Build history of the part. All positions in model axes, mm. Face numbers are marked on the shaded views. A direction names the side the tool comes from. Coordinates: 2 decimals unless noted, no trailing zeros. Loops run counter-clockwise (first coordinate to the right, second up) from the corner with the lowest first, then second, coordinate; pieces in that order, holes last.
Item 1: 3-axis set-ups, long thin cutter, end or side, ignore diameter. For the marked faces 1, 2 and 3: which of +Z, -Z, +X, -X, +Y, -Y reach the whole face in a straight line?
Item 2: Cut at B-B (x = 59). List the corners of the cut face in (y, z).
Item 3: Cut at C-C (y = -60). List the corners of the cut face in (x, z), and give its area (3 significant figures).
Item 4: Cut at A-A (z = 22). List the corners of the cut face in (x, y).
Item 5: Flat gauge pins, fed straight in: pin 1 (16.5 mm diameter, centred on x = 82, y = 57, fed in from +Z); pin 2 (9 mm diameter, centred on x = -5.5, z = 12, fed in from +Y); pin 3 (15 mm diameter, centred on x = 54, z = 12, fed in from -Y). Where does each tip first touch, or does it go through?
Item 6: Drill centre lines: line 1 along Y through (x, z) = (136, 21); line 2 along Z through (x, y) = (-18, 33.5). Where is each one in solid material? Low to high.
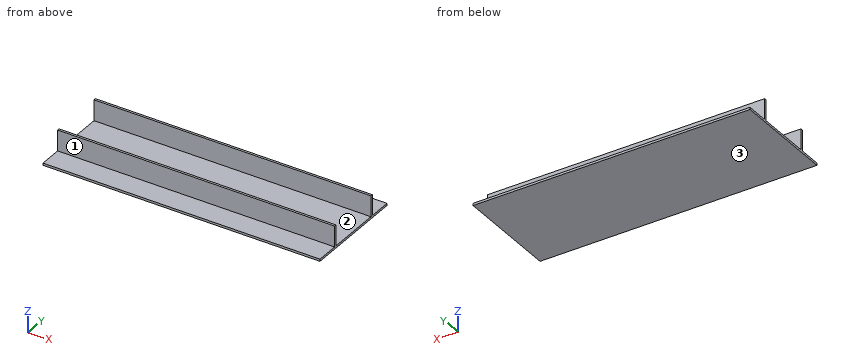
from build123d import *

# Parameters (mm, degrees)
F0_W     = 400
F0_H     = 150
F1_DEPTH = 1.5875
F2_W     = 400
F2_H     = 3.175
F3_DEPTH = 30


with BuildPart() as f1:
    # F0 (on Top) → F1 (new body, symmetric)
    with BuildSketch(Plane.XY):
        Rectangle(F0_W, F0_H)
    extrude(amount=F1_DEPTH, both=True)

    # F2 (on face) → F3 (join)
    with BuildSketch(Plane.XY.offset(1.5875)):
        with Locations((0, 40.618111515)):
            Rectangle(F2_W, F2_H)
    extrude(amount=F3_DEPTH)

    # F4: F1 across plane


with BuildPart() as f1_1:
    add(f1.part)
    add(f1.part.mirror(Plane.XZ))


solid = f1_1.part
Filled sheet:
1. face 1: +Z, +X, -X, -Y
1. face 2: +Z, +X, -X
1. face 3: -Z, +X, -X, +Y, -Y
2. outline: (-75, -1.59) - (75, -1.59) - (75, 1.59) - (42.21, 1.59) - (42.21, 31.59) - (39.03, 31.59) - (39.03, 1.59) - (-39.03, 1.59) - (-39.03, 31.59) - (-42.21, 31.59) - (-42.21, 1.59) - (-75, 1.59) - close
3. outline: (-200, -1.59) - (200, -1.59) - (200, 1.59) - (-200, 1.59) - close
3. area: 1,270 mm2
4. outline: (-200, -42.21) - (200, -42.21) - (200, -39.03) - (-200, -39.03) - close; (-200, 39.03) - (200, 39.03) - (200, 42.21) - (-200, 42.21) - close
5. pin 1: stops at z = 1.59
5. pin 2: stops at y = 42.21
5. pin 3: stops at y = -42.21
6. line 1: y = -42.21 to -39.03, 39.03 to 42.21
6. line 2: z = -1.59 to 1.59
